Check sheet for the drawn part. Datum: minimum x, y, z corner. Units: mm. Give positions to 0.01 mm unless a question says otherwise; leave off trailing zeros. Write each loop counter-clockwise with the first axis right and the second up, starting at its lowest first coordinate (ties: lowest second). Pieces come first, ordered by that corner, then holes. Notation, with made-up numbers: (81.25, 46) -> (94.25, 46) arc R15 ccw to (94.25, 72) -> close; hole circle Ø1 at (21.5, 48.25). An arc over 180 degrees is marked (long way). Write item = value, one per line. Start each with the question number.
1. Thickness scan on line 1 along X through (y, z) = (3.5, 0.55); line 2 along X through (y, z) = (3.5, 4.6). Record the ranges inside material, lowest first.
2. Cross-section at A-A, the plane y = 2.75. Record the cut outline in (x, z).
3. Depth check by flat-ended pin: P1, Ø0.6, axis at y = 2, z = 3, coming from the -X side; P2, Ø1, axis at y = 4.5, z = 0.5, coming from the +X side; P3, Ø0.6, axis at y = 2.5, z = 4.5, coming from the -X side. Enter the tip coordinate at first touch or a pass-through.
4. Mould release check, pull along Z, two halves, no side actions. Record for the marked faces 1, 2 and 3: pulls with the +Z half, pulls with the -Z half, needs draft (parallel to the pull), parting line crosses it, or undercut.
5. Cross-section at B-B, the plane z = 4.45. Record the cut outline in (x, y).
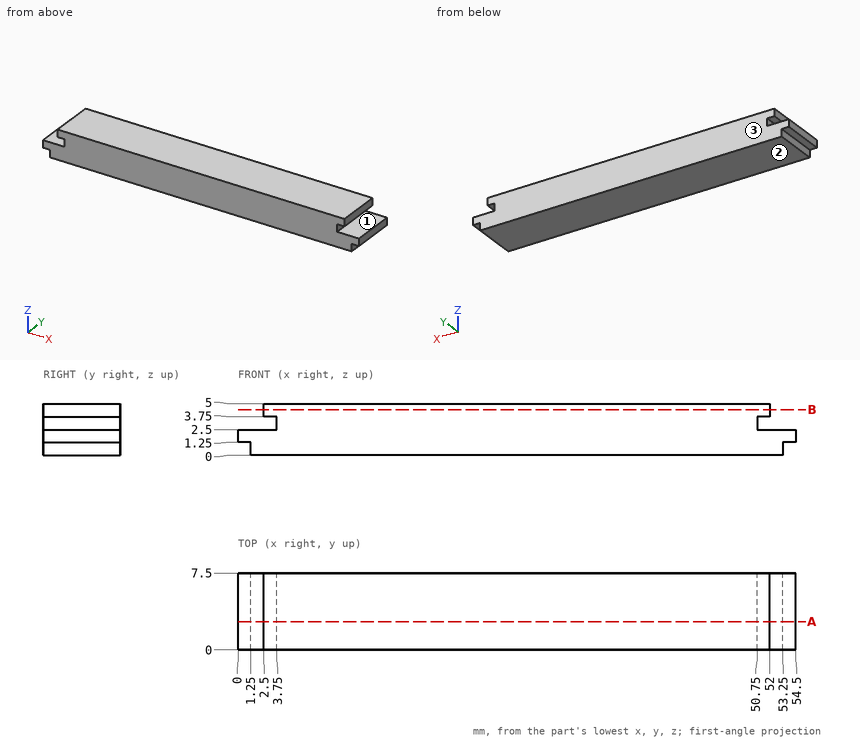
Answers:
q1.line_1 = 1.25 to 53.25
q1.line_2 = 2.5 to 52
q2.outline = (0, 1.25) -> (1.25, 1.25) -> (1.25, 0) -> (53.25, 0) -> (53.25, 1.25) -> (54.5, 1.25) -> (54.5, 2.5) -> (50.75, 2.5) -> (50.75, 3.75) -> (52, 3.75) -> (52, 5) -> (2.5, 5) -> (2.5, 3.75) -> (3.75, 3.75) -> (3.75, 2.5) -> (0, 2.5) -> close
q3.P1 = 3.75
q3.P2 = 53.25
q3.P3 = 2.5
q4.face_1 = undercut
q4.face_2 = pulls with the -Z half
q4.face_3 = needs draft
q5.outline = (2.5, 0) -> (52, 0) -> (52, 7.5) -> (2.5, 7.5) -> close
